Part model, mm, in its own coordinate system. Face numbers are marked on the shaded views. A direction names the side the tool comes from. Coordinates: 2 decimals unless noted, no trailing zeros. Order: outer loops, then holes, each group sorted by start corner. A loop starts at its lowest first (then second) coordinate and runs counter-clockwise, first axis right, second up. Notation, with made-up numbers: M 68.25,0.25 L 112.25,0.25 A13 ccw 112.25,9.25 Z; hole C 3.5,72.5 d11. An arc over 180 degrees is marked long. Write item = value, one per line. Start each with the question number.
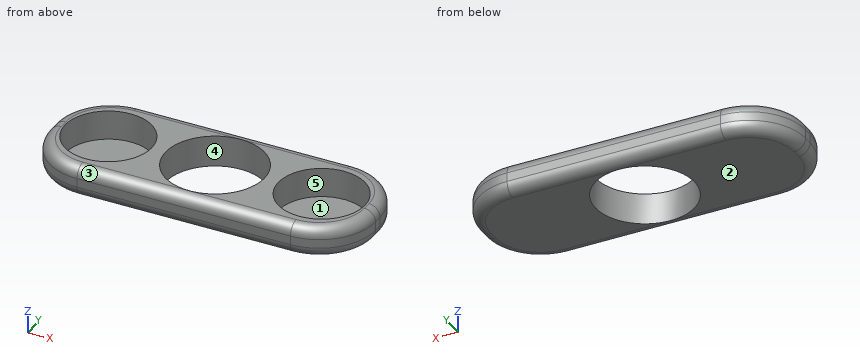
from build123d import *

# Parameters (mm, degrees)
F0_R     = 9.725
F0_R_2   = 11.1
F1_DEPTH = 7
F2_R     = 2.5
F3_R     = 9.75
F4_DEPTH = 0.4


with BuildPart() as f1:
    # F0 (on Top) → F1 (new body)
    with BuildSketch(Plane.XY):
        with BuildLine():
            Line((24, 13.625), (-24, 13.625))
            ThreePointArc((-24, 13.625), (-32.927223, 9.927223), (-36.625, 1))
            Line((-36.625, 1), (-36.625, -1))
            ThreePointArc((-36.625, -1), (-32.927223, -9.927223), (-24, -13.625))
            Line((-24, -13.625), (24, -13.625))
            ThreePointArc((24, -13.625), (32.927223, -9.927223), (36.625, -1))
            Line((36.625, -1), (36.625, 1))
            ThreePointArc((36.625, 1), (32.927223, 9.927223), (24, 13.625))
        make_face()
        with Locations((-24, 0)):
            Circle(F0_R, mode=Mode.SUBTRACT)
        Circle(F0_R_2, mode=Mode.SUBTRACT)
        with Locations((24, 0)):
            Circle(F0_R, mode=Mode.SUBTRACT)
    extrude(amount=F1_DEPTH)

    # F2
    f2_edges = [f1.edges().sort_by_distance(p)[0] for p in [
        (0, -13.625, 7),
        (0, -13.625, 0),
    ]]
    fillet(f2_edges, radius=F2_R)

    # F3 (on Top) → F4 (join)
    with BuildSketch(Plane.XY):
        with Locations((-24, 0)):
            Circle(F3_R)
        with Locations((24, 0)):
            Circle(F3_R)
    extrude(amount=F4_DEPTH)


solid = f1.part
Item 1: Cut at C-C, the plane z = 1.25. Write the cut outline in (x, y) (3 decimals), and give its area (3 significant figures).
Item 2: Cut at D-D, the plane z = 5.5. Write the cut outline in (x, y) (3 decimals).
Item 3: 3-axis set-ups, long thin cutter, end or side, ignore diameter. For the marked faces 4 and 5: which of +Z, -Z, +X, -X, +Y, -Y reach the whole face in a straight line?
Item 4: Cut at A-A, the plane y = 0. Write the cut outline in (x, z) (3 decimals).
Item 5: Cut at B-B, the plane x = 0. Write the cut outline in (y, z) (3 decimals), and give its area (3 significant figures).
Item 6: Pull direction Y, two halves, no side cores. Call the marked faces 1, 2 and 3: pulls with the +Y half, pulls with the -Y half, needs draft (parallel to the pull), parting line crosses it, or undercut.
Item 7: Wall check: line 1 along X through (y, z) = (-8.5, 5.75) (3 decimals); line 2 along X through (y, z) = (-4, 3.25); line 3 along Y through (x, z) = (0, 3) (3 decimals). Give the ranges that are in metal, low to high. Write a range as [from, to].
Item 8: Flat gauge pin, fed straight in: pin 1 (6 mm diameter, centred on x = -25, y = -4, fed in from +Z). Where does the tip first touch, or does it go through?
Filled sheet:
q1.outline = M -36.29,-1 A12.29 ccw -24,-13.29 L 24,-13.29 A12.29 ccw 36.29,-1 L 36.29,1 A12.29 ccw 24,13.29 L -24,13.29 A12.29 ccw -36.29,1 Z; hole C -24,0 d19.45; hole C 0,0 d22.2; hole C 24,0 d19.45
q1.area = 818 mm2
q2.outline = M -36.416,-1 A12.416 ccw -24,-13.416 L 24,-13.416 A12.416 ccw 36.416,-1 L 36.416,1 A12.416 ccw 24,13.416 L -24,13.416 A12.416 ccw -36.416,1 Z; hole C -24,0 d19.45; hole C 0,0 d22.2; hole C 24,0 d19.45
q3.face_4 = +Z, -Z
q3.face_5 = +Z
q4.outline = M -36.625,2.5 A2.5 ccw -34.125,0 L -11.1,0 L -11.1,7 L -14.275,7 L -14.275,0.4 L -33.725,0.4 L -33.725,7 L -34.125,7 A2.5 ccw -36.625,4.5 Z; M 11.1,0 L 34.125,0 A2.5 ccw 36.625,2.5 L 36.625,4.5 A2.5 ccw 34.125,7 L 33.725,7 L 33.725,0.4 L 14.275,0.4 L 14.275,7 L 11.1,7 Z
q5.outline = M -13.625,2.5 A2.5 ccw -11.125,0 L -11.1,0 L -11.1,7 L -11.125,7 A2.5 ccw -13.625,4.5 Z; M 11.1,0 L 11.125,0 A2.5 ccw 13.625,2.5 L 13.625,4.5 A2.5 ccw 11.125,7 L 11.1,7 Z
q5.area = 30.0 mm2
q6.face_1 = undercut
q6.face_2 = needs draft
q6.face_3 = pulls with the -Y half
q7.line_1 = [-33.736, -28.725], [-19.275, -7.139], [7.139, 19.275], [28.725, 33.736]
q7.line_2 = [-36.26, -32.86], [-15.14, -10.35], [10.35, 15.14], [32.86, 36.26]
q7.line_3 = [-13.625, -11.1], [11.1, 13.625]
q8.pin_1 = 0.4
